Here's how the part is built. I have some questions about the finished solid (model axes, mm). Face numbers are marked on the shaded views. A direction names the side the tool comes from. Round coordinates to 2 decimals unless told otherwise and drop trailing zeros. Order: outer loops, then holes, each group sorted by start corner. A loop starts at its lowest first (then second) coordinate and runs counter-clockwise, first axis right, second up. Notation, with made-up numbers: (46, -3) -> (100, -3) arc R26 ccw to (100, 19) -> close; hole circle Ø5 at (59, 41). An arc over 180 degrees is marked (long way). Use a Markdown table: item, result. Add a question column.
(1) I want a section at C-C, the plane x = 24. Please give me the cut outline in (y, z).
(2) I'm going to push flat-ended pins straight in: P1, Ø6, axis at y = 19.5, z = -10.5, coming from the -X side; P2, Ø10, axis at y = 19, z = -4.5, coming from the -X side; P3, Ø4.5, axis at y = 21, z = -9.5, coming from the +X side. Where does each tip first touch, or does it pass through?
(3) On a 3-axis mill with a long thin cutter (end or side, diameter ignored), from which of +Z, -Z, +X, -X, +Y, -Y can I reach the whole of each face in a straight line? I mean the marked faces 1, 2 and 3. Say none if no direction works.
(4) If I drill on probe 1 along Y at (x, z) = (19, -7); probe 2 along X at (y, z) = (27.5, 8); probe 3 along Z at (x, y) = (46.5, 16.5), over which ranges is the centre line in solid material (lowest first)?
(5) I want a section at D-D, the plane y = 13. Please give me the cut outline in (x, z), then the cut area to 3 significant figures.
(6) I want a section at B-B, the plane z = -5.5. Please give me the cut outline in (x, y), then the cut area to 3 significant figures.
(7) I want a section at A-A, the plane y = 29.5. Please give me the cut outline in (x, z).
from build123d import *

# Parameters (mm, degrees)
BOSS_EXTRUDE1_DEPTH = 15.5
BOSS_EXTRUDE2_DEPTH = 4
SKETCH3_W           = 9
SKETCH3_H           = 13
BOSS_EXTRUDE3_DEPTH = 42


with BuildPart() as part:
    # Sketch1 → Boss-Extrude1 (new, symmetric)
    with BuildSketch(Plane.XY):
        Polygon((0, 0), (0, 12), (62, 12), (62, 42), (76, 42), (76, 0), align=None)
    extrude(amount=BOSS_EXTRUDE1_DEPTH, both=True)

    # Sketch2 → Boss-Extrude2 (add, symmetric)
    with BuildSketch(Plane.XY):
        Polygon((8, 12), (62, 42), (62, 12), align=None)
    extrude(amount=BOSS_EXTRUDE2_DEPTH, both=True)

    # Sketch3 → Boss-Extrude3 (add, through all)
    with BuildSketch(Plane(origin=(0, 42, 0), x_dir=(1, 0, 0), z_dir=(0, 1, 0))):
        with Locations((80.5, 0)):
            Rectangle(SKETCH3_W, SKETCH3_H)
    extrude(amount=-BOSS_EXTRUDE3_DEPTH)


solid = part.part
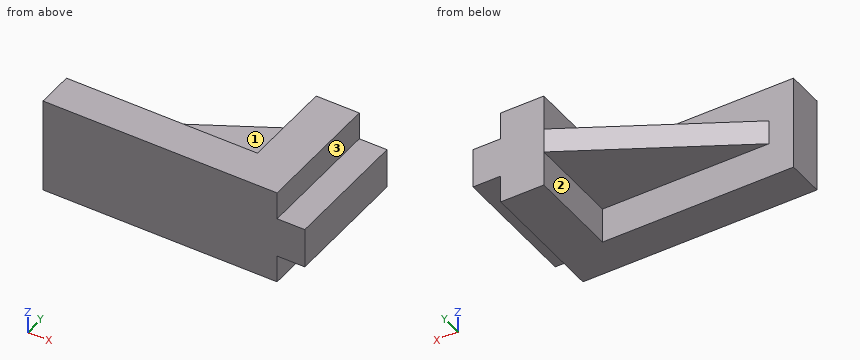
Taken from the geometry:
| question | item | result |
|---|---|---|
| 1 | outline | (0, -15.5) -> (12, -15.5) -> (12, -4) -> (20.89, -4) -> (20.89, 4) -> (12, 4) -> (12, 15.5) -> (0, 15.5) -> close |
| 2 | P1 | stops at x = 62 |
| 2 | P2 | stops at x = 11.65 |
| 2 | P3 | stops at x = 76 |
| 3 | face 1 | +Z, -X, +Y |
| 3 | face 2 | -Z, -X, +Y |
| 3 | face 3 | +Z, +X, +Y, -Y |
| 4 | probe 1 | y = 0 to 12 |
| 4 | probe 2 | x = 62 to 76 |
| 4 | probe 3 | z = -4 to 4 |
| 5 | outline | (9.8, -4) -> (62, -4) -> (62, -15.5) -> (76, -15.5) -> (76, -6.5) -> (85, -6.5) -> (85, 6.5) -> (76, 6.5) -> (76, 15.5) -> (62, 15.5) -> (62, 4) -> (9.8, 4) -> close |
| 5 | area | 969 mm2 |
| 6 | outline | (0, 0) -> (85, 0) -> (85, 42) -> (62, 42) -> (62, 12) -> (0, 12) -> close |
| 6 | area | 1,710 mm2 |
| 7 | outline | (39.5, -4) -> (62, -4) -> (62, -15.5) -> (76, -15.5) -> (76, -6.5) -> (85, -6.5) -> (85, 6.5) -> (76, 6.5) -> (76, 15.5) -> (62, 15.5) -> (62, 4) -> (39.5, 4) -> close |
